Can you work these out from the model? Positions are in its coordinate system, mm. Round coordinates to 2 decimals unless told otherwise and drop trailing zeros. Loops run counter-clockwise (first coordinate to the right, second up) from the corner with the lowest first, then second, coordinate; pieces in that order, holes last. Notation, with made-up numbers: (-37, -20.5) - (-17, -20.5) arc R18 ccw to (-17, 7.5) - close; hole circle Ø5 at (34, -17). An arc over 180 degrees is marked (long way). Answer as CSV lines item,"result".
```python
from build123d import *

# Parameters (mm, degrees)
F0_R     = 45
F1_DEPTH = 3
F0_R_2   = 49
F3_DEPTH = 3
F5_R     = 28
F6_DEPTH = 3
F5_R_2   = 31
F8_DEPTH = 3


with BuildPart() as f1:
    # F0 (on Top) → F1 (new body)
    with BuildSketch(Plane.XY):
        Polygon((38.83281573, -28.21369211), (48, 0), (38.83281573, 28.21369211), (14.83281573, 45.6507127822), (-14.83281573, 45.6507127822), (-38.83281573, 28.21369211), (-48, 0), (-38.83281573, -28.21369211), (-14.83281573, -45.6507127822), (14.83281573, -45.6507127822), align=None)
        Circle(F0_R, mode=Mode.SUBTRACT)
    extrude(amount=-F1_DEPTH)

    # F0 (on Top) → F3 (join)
    with BuildSketch(Plane.XY):
        Circle(F0_R_2)
        Polygon((38.83281573, 28.21369211), (48, 0), (38.83281573, -28.21369211), (14.83281573, -45.6507127822), (-14.83281573, -45.6507127822), (-38.83281573, -28.21369211), (-48, 0), (-38.83281573, 28.21369211), (-14.83281573, 45.6507127822), (14.83281573, 45.6507127822), align=None, mode=Mode.SUBTRACT)
    extrude(amount=-F3_DEPTH)



with BuildPart() as f6:
    # F5 (on offset) → F6 (new body)
    with BuildSketch(Plane.XY.offset(-40)):
        Polygon((24.2705098312, -17.6335575688), (30, 0), (24.2705098312, 17.6335575688), (9.2705098312, 28.5316954889), (-9.2705098312, 28.5316954889), (-24.2705098312, 17.6335575688), (-30, 0), (-24.2705098312, -17.6335575688), (-9.2705098312, -28.5316954889), (9.2705098312, -28.5316954889), align=None)
        Circle(F5_R, mode=Mode.SUBTRACT)
    extrude(amount=-F6_DEPTH)

    # F5 (on offset) → F8 (join)
    with BuildSketch(Plane.XY.offset(-40)):
        Circle(F5_R_2)
        Polygon((24.2705098312, 17.6335575688), (30, 0), (24.2705098312, -17.6335575688), (9.2705098312, -28.5316954889), (-9.2705098312, -28.5316954889), (-24.2705098312, -17.6335575688), (-30, 0), (-24.2705098312, 17.6335575688), (-9.2705098312, 28.5316954889), (9.2705098312, 28.5316954889), align=None, mode=Mode.SUBTRACT)
    extrude(amount=-F8_DEPTH)


with BuildPart() as f1_1:
    add(f1.part)

    add(f6.part)  # F9 merges F6
    # F2 (on face) → F9 section 0
    with BuildSketch(Plane(origin=(0, 0, -3), x_dir=(1, 0, 0), z_dir=(0, 0, -1))):
        with BuildLine():
            ThreePointArc((-47.0729490169, 2.8531695489), (-51, 0), (-47.0729490169, -2.8531695489))
            Line((-47.0729490169, -2.8531695489), (-48, 0))
            Line((-48, 0), (-47.0729490169, 2.8531695489))
        make_face()
    # F7 (on face) → F9 section 1
    with BuildSketch(Plane.XY.offset(-40)):
        with BuildLine():
            ThreePointArc((-29.3819660113, 1.9021130326), (-32, 0), (-29.3819660113, -1.9021130326))
            Line((-29.3819660113, -1.9021130326), (-30, 0))
            Line((-30, 0), (-29.3819660113, 1.9021130326))
        make_face()
    loft()

    # F7 (on face) → F10 section 0
    with BuildSketch(Plane.XY.offset(-40)):
        with BuildLine():
            ThreePointArc((-24.88854382, -15.7314445362), (-25.88854382, -18.8091280734), (-22.6524758425, -18.8091280734))
            Line((-22.6524758425, -18.8091280734), (-24.2705098312, -17.6335575688))
            Line((-24.2705098312, -17.6335575688), (-24.88854382, -15.7314445362))
        make_face()
    # F2 (on face) → F10 section 1
    with BuildSketch(Plane(origin=(0, 0, -3), x_dir=(1, 0, 0), z_dir=(0, 0, -1))):
        with BuildLine():
            ThreePointArc((-36.4057647469, 29.9770478669), (-41.2598667131, 29.9770478669), (-39.7598667131, 25.3605225612))
            Line((-39.7598667131, 25.3605225612), (-38.83281573, 28.21369211))
            Line((-38.83281573, 28.21369211), (-36.4057647469, 29.9770478669))
        make_face()
    loft()

    # F2 (on face) → F11 section 0
    with BuildSketch(Plane(origin=(0, 0, -3), x_dir=(1, 0, 0), z_dir=(0, 0, -1))):
        with BuildLine():
            ThreePointArc((-11.83281573, 45.6507127822), (-15.7598667131, 48.5038823311), (-17.2598667131, 43.8873570253))
            Line((-17.2598667131, 43.8873570253), (-14.83281573, 45.6507127822))
            Line((-14.83281573, 45.6507127822), (-11.83281573, 45.6507127822))
        make_face()
    # F7 (on face) → F11 section 1
    with BuildSketch(Plane.XY.offset(-40)):
        with BuildLine():
            Line((-9.2705098312, -28.5316954889), (-10.88854382, -27.3561249843))
            ThreePointArc((-10.88854382, -27.3561249843), (-9.88854382, -30.4338085214), (-7.2705098312, -28.5316954889))
            Line((-7.2705098312, -28.5316954889), (-9.2705098312, -28.5316954889))
        make_face()
    loft()

    # F7 (on face) → F12 section 0
    with BuildSketch(Plane.XY.offset(-40)):
        with BuildLine():
            Line((9.2705098312, -28.5316954889), (7.2705098312, -28.5316954889))
            ThreePointArc((7.2705098312, -28.5316954889), (9.2705098312, -30.5316954889), (11.2705098312, -28.5316954889))
            ThreePointArc((11.2705098312, -28.5316954889), (11.1726228638, -27.9136615001), (10.88854382, -27.3561249843))
            Line((10.88854382, -27.3561249843), (9.2705098312, -28.5316954889))
        make_face()
    # F2 (on face) → F12 section 1
    with BuildSketch(Plane(origin=(0, 0, -3), x_dir=(1, 0, 0), z_dir=(0, 0, -1))):
        with BuildLine():
            ThreePointArc((17.83281573, 45.6507127822), (14.83281573, 48.6507127822), (11.83281573, 45.6507127822))
            Line((11.83281573, 45.6507127822), (14.83281573, 45.6507127822))
            Line((14.83281573, 45.6507127822), (17.2598667131, 43.8873570253))
            ThreePointArc((17.2598667131, 43.8873570253), (17.6859852789, 44.723661799), (17.83281573, 45.6507127822))
        make_face()
    loft()

    # F2 (on face) → F13 section 0
    with BuildSketch(Plane(origin=(0, 0, -3), x_dir=(1, 0, 0), z_dir=(0, 0, -1))):
        with BuildLine():
            ThreePointArc((41.83281573, 28.21369211), (39.7598667131, 31.0668616589), (36.4057647469, 29.9770478669))
            Line((36.4057647469, 29.9770478669), (38.83281573, 28.21369211))
            Line((38.83281573, 28.21369211), (39.7598667131, 25.3605225612))
            ThreePointArc((39.7598667131, 25.3605225612), (41.2598667131, 26.4503363532), (41.83281573, 28.21369211))
        make_face()
    # F7 (on face) → F13 section 1
    with BuildSketch(Plane.XY.offset(-40)):
        with BuildLine():
            Line((24.2705098312, -17.6335575688), (22.6524758425, -18.8091280734))
            ThreePointArc((22.6524758425, -18.8091280734), (24.88854382, -19.5356706014), (26.2705098312, -17.6335575688))
            ThreePointArc((26.2705098312, -17.6335575688), (25.88854382, -16.4579870642), (24.88854382, -15.7314445362))
            Line((24.88854382, -15.7314445362), (24.2705098312, -17.6335575688))
        make_face()
    loft()

    # F7 (on face) → F14 section 0
    with BuildSketch(Plane.XY.offset(-40)):
        with BuildLine():
            Line((30, 0), (29.3819660113, -1.9021130326))
            ThreePointArc((29.3819660113, -1.9021130326), (31.1755705046, -1.6180339887), (32, 0))
            ThreePointArc((32, 0), (31.1755705046, 1.6180339887), (29.3819660113, 1.9021130326))
            Line((29.3819660113, 1.9021130326), (30, 0))
        make_face()
    # F2 (on face) → F14 section 1
    with BuildSketch(Plane(origin=(0, 0, -3), x_dir=(1, 0, 0), z_dir=(0, 0, -1))):
        with BuildLine():
            Line((48, 0), (47.0729490169, -2.8531695489))
            ThreePointArc((47.0729490169, -2.8531695489), (49.7633557569, -2.4270509831), (51, 0))
            ThreePointArc((51, 0), (49.7633557569, 2.4270509831), (47.0729490169, 2.8531695489))
            Line((47.0729490169, 2.8531695489), (48, 0))
        make_face()
    loft()

    # F2 (on face) → F15 section 0
    with BuildSketch(Plane(origin=(0, 0, -3), x_dir=(1, 0, 0), z_dir=(0, 0, -1))):
        with BuildLine():
            Line((38.83281573, -28.21369211), (36.4057647469, -29.9770478669))
            ThreePointArc((36.4057647469, -29.9770478669), (39.7598667131, -31.0668616589), (41.83281573, -28.21369211))
            ThreePointArc((41.83281573, -28.21369211), (41.2598667131, -26.4503363532), (39.7598667131, -25.3605225612))
            Line((39.7598667131, -25.3605225612), (38.83281573, -28.21369211))
        make_face()
    # F7 (on face) → F15 section 1
    with BuildSketch(Plane.XY.offset(-40)):
        with BuildLine():
            ThreePointArc((26.2705098312, 17.6335575688), (24.88854382, 19.5356706014), (22.6524758425, 18.8091280734))
            Line((22.6524758425, 18.8091280734), (24.2705098312, 17.6335575688))
            Line((24.2705098312, 17.6335575688), (24.88854382, 15.7314445362))
            ThreePointArc((24.88854382, 15.7314445362), (25.88854382, 16.4579870642), (26.2705098312, 17.6335575688))
        make_face()
    loft()

    # F7 (on face) → F16 section 0
    with BuildSketch(Plane.XY.offset(-40)):
        with BuildLine():
            ThreePointArc((11.2705098312, 28.5316954889), (9.2705098312, 30.5316954889), (7.2705098312, 28.5316954889))
            Line((7.2705098312, 28.5316954889), (9.2705098312, 28.5316954889))
            Line((9.2705098312, 28.5316954889), (10.88854382, 27.3561249843))
            ThreePointArc((10.88854382, 27.3561249843), (11.1726228638, 27.9136615001), (11.2705098312, 28.5316954889))
        make_face()
    # F2 (on face) → F16 section 1
    with BuildSketch(Plane(origin=(0, 0, -3), x_dir=(1, 0, 0), z_dir=(0, 0, -1))):
        with BuildLine():
            Line((14.83281573, -45.6507127822), (11.83281573, -45.6507127822))
            ThreePointArc((11.83281573, -45.6507127822), (14.83281573, -48.6507127822), (17.83281573, -45.6507127822))
            ThreePointArc((17.83281573, -45.6507127822), (17.6859852789, -44.723661799), (17.2598667131, -43.8873570253))
            Line((17.2598667131, -43.8873570253), (14.83281573, -45.6507127822))
        make_face()
    loft()

    # F2 (on face) → F17 section 0
    with BuildSketch(Plane(origin=(0, 0, -3), x_dir=(1, 0, 0), z_dir=(0, 0, -1))):
        with BuildLine():
            Line((-14.83281573, -45.6507127822), (-17.2598667131, -43.8873570253))
            ThreePointArc((-17.2598667131, -43.8873570253), (-15.7598667131, -48.5038823311), (-11.83281573, -45.6507127822))
            Line((-11.83281573, -45.6507127822), (-14.83281573, -45.6507127822))
        make_face()
    # F7 (on face) → F17 section 1
    with BuildSketch(Plane.XY.offset(-40)):
        with BuildLine():
            ThreePointArc((-7.2705098312, 28.5316954889), (-9.88854382, 30.4338085214), (-10.88854382, 27.3561249843))
            Line((-10.88854382, 27.3561249843), (-9.2705098312, 28.5316954889))
            Line((-9.2705098312, 28.5316954889), (-7.2705098312, 28.5316954889))
        make_face()
    loft()

    # F7 (on face) → F18 section 0
    with BuildSketch(Plane.XY.offset(-40)):
        with BuildLine():
            ThreePointArc((-22.6524758425, 18.8091280734), (-25.88854382, 18.8091280734), (-24.88854382, 15.7314445362))
            Line((-24.88854382, 15.7314445362), (-24.2705098312, 17.6335575688))
            Line((-24.2705098312, 17.6335575688), (-22.6524758425, 18.8091280734))
        make_face()
    # F2 (on face) → F18 section 1
    with BuildSketch(Plane(origin=(0, 0, -3), x_dir=(1, 0, 0), z_dir=(0, 0, -1))):
        with BuildLine():
            ThreePointArc((-39.7598667131, -25.3605225612), (-41.2598667131, -29.9770478669), (-36.4057647469, -29.9770478669))
            Line((-36.4057647469, -29.9770478669), (-38.83281573, -28.21369211))
            Line((-38.83281573, -28.21369211), (-39.7598667131, -25.3605225612))
        make_face()
    loft()


solid = f1_1.part
```
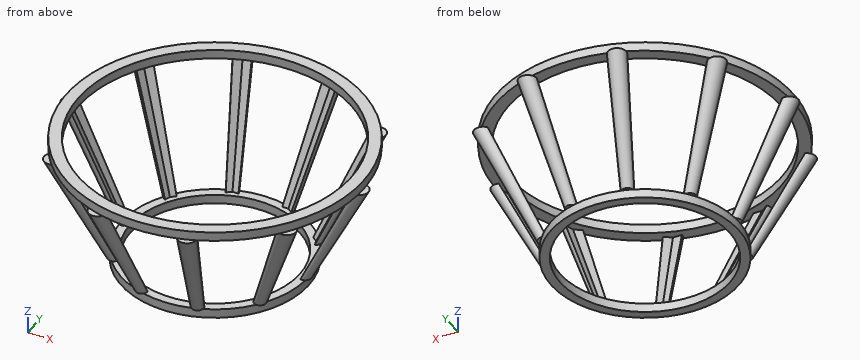
Q1. I'm going to push flat-ended pins straight in: pin 1 Ø1.2 at (x, y) = (-40.5, -28.5) entering from +Z; pin 2 Ø8 at (x, y) = (-9, 36.5) entering from -Z; pin 3 Ø1 at (x, y) = (-50, 1) entering from +Z; pin 4 Ø0.8 at (x, y) = (31.5, 0) entering from -Z. Where does each tip first touch, or does it pass through?
Checks:
pin 1,"z = 0"
pin 2,"z = -35.85"
pin 3,"z = -3"
pin 4,"z = -40"
Q2. Imagine slicing it at B-B (x = 0). Write out the boundary of the cut face in (y, z), then the cut area to 3 significant figures.
Checks:
outline,"(-49, -3) - (-45, -3) - (-45, 0) - (-49, 0) - close; (-31, -43) - (-28, -43) - (-28, -40) - (-31, -40) - close; (28, -43) - (31, -43) - (31, -40) - (28, -40) - close; (45, -3) - (49, -3) - (49, 0) - (45, 0) - close"
area,"42.0 mm²"
Q3. Imagine slicing it at A-A (y = 6). Write out the boundary of the cut face in (x, z), then the cut area to 3 significant figures.
Checks:
outline,"(-48.63, -3) - (-44.6, -3) - (-44.6, 0) - (-48.63, 0) - close; (-30.41, -43) - (-27.35, -43) - (-27.35, -40) - (-30.41, -40) - close; (27.35, -43) - (30.41, -43) - (30.41, -40) - (27.35, -40) - close; (44.6, -3) - (48.63, -3) - (48.63, 0) - (44.6, 0) - close"
area,"42.6 mm²"
Q4. If I drill on line 1 along Y through (x, z) = (0, -2.05); line 2 along Y through (x, z) = (0, -42.1); line 3 along X through (y, z) = (1, -23), over which ranges is the centre line in solid material (lowest first)? Write a range as [from, to].
Checks:
line 1,"[-49, -45], [45, 49]"
line 2,"[-31, -28], [28, 31]"
line 3,"[-40.52, -37.95], [37.95, 40.52]"
Q5. Imagine slicing it at C-C (z = -36). Count the separate pieces of the cut face and the enclosed holes in it, then the cut area to 3 significant figures.
Checks:
separate pieces,"10"
enclosed holes,"0"
area,"83.8 mm²"
